Geometry: see drawing. Coordinates: mm, zero at the bounding-box minimum. A direction names the side the tool comes from. Coordinates: 2 decimals unless noted, no trailing zeros. Order: outer loops, then holes, each group sorted by start corner. A loop starts at its lowest first (then second) coordinate and runs counter-clockwise, first axis right, second up. Notation, with made-up numbers: (-31.75, 85.25) - (-13.75, 85.25) arc R13 ccw to (-13.75, 90.25) - close; hole circle Ø11 at (-4, 79). An arc over 180 degrees is marked (long way). Use a Markdown table: item, result. Add a question column.
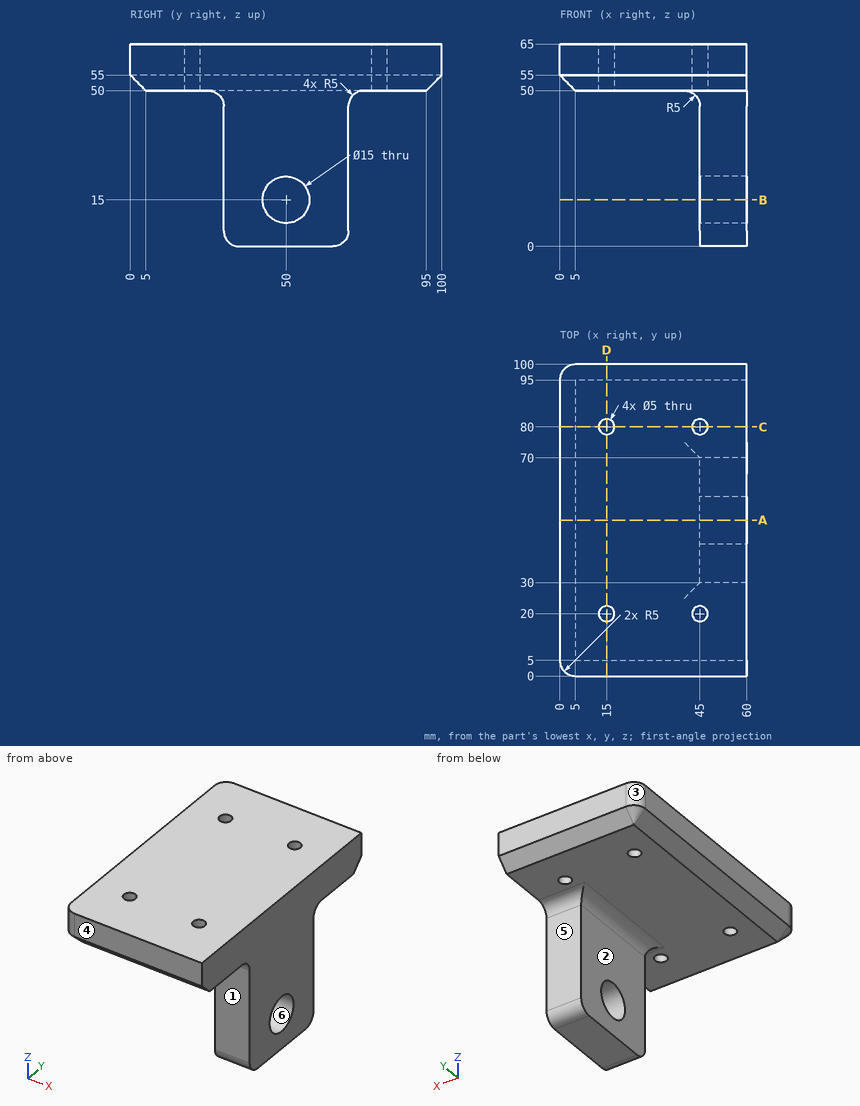
1) Cut plane D-D (x = 15). Return the cut outline in (y, z).
2) Cut plane C-C (y = 80). Return the cut outline in (x, z).
3) Cut plane B-B (z = 15). Return the cut outline in (x, y), and give its area (3 significant figures).
4) Material intervals for L1, parallel to Y at x = 15, z = 56.75; L2, parallel to Z at x = 56, y = 14.5; L3, parallel to Y at x = 49, z = 33.5, sorted ascending.
5) Reachability of the marked faces 1, 2 and 3 from +Z, -Z, +X, -X, +Y, -Y: full face, straight path, thin tool, end or side. Return the list, or none.
6) Contact query for flat-ended pins moving along their axis: P1, Ø2, axis at x = 46.5, y = 66.5, coming from the -Z side; P2, Ø4.5, axis at x = 49.5, z = 21.5, coming from the +Y side; P3, Ø1, axis at y = 58.5, z = 24, coming from the -X side; P4, Ø17, axis at y = 50, z = 15, coming from the +X side. Output: stop coordinate, or through.
7) Cut plane A-A (y = 50). Return the cut outline in (x, z), and give its area (3 significant figures).
8) Pull-direction query (Y, two-part tool) for the marked faces 4, 5 and 6; classes: pulls with the +Y half, pulls with the -Y half, needs draft (parallel to the pull), parting line crosses it, or undercut.
Computed:
| question | item | result |
|---|---|---|
| 1 | outline | (0, 55) - (5, 50) - (17.5, 50) - (17.5, 65) - (0, 65) - close; (22.5, 50) - (77.5, 50) - (77.5, 65) - (22.5, 65) - close; (82.5, 50) - (95, 50) - (100, 55) - (100, 65) - (82.5, 65) - close |
| 2 | outline | (0, 55) - (5, 50) - (12.5, 50) - (12.5, 65) - (0, 65) - close; (17.5, 50) - (42.5, 50) - (42.5, 65) - (17.5, 65) - close; (47.5, 50) - (60, 50) - (60, 65) - (47.5, 65) - close |
| 3 | outline | (45, 30) - (60, 30) - (60, 42.5) - (45, 42.5) - close; (45, 57.5) - (60, 57.5) - (60, 70) - (45, 70) - close |
| 3 | area | 375 mm2 |
| 4 | L1 | y = 0 to 17.5, 22.5 to 77.5, 82.5 to 100 |
| 4 | L2 | z = 50 to 65 |
| 4 | L3 | y = 30 to 70 |
| 5 | face 1 | -Z, +X, -X, -Y |
| 5 | face 2 | -Z, -X, +Y, -Y |
| 5 | face 3 | +Z, -Z, -X, +Y |
| 6 | P1 | stops at z = 0.03 |
| 6 | P2 | stops at y = 70 |
| 6 | P3 | stops at x = 45 |
| 6 | P4 | stops at x = 60 |
| 7 | outline | (0, 55) - (5, 50) - (40, 50) arc R5 cw to (45, 45) - (45, 22.5) - (60, 22.5) - (60, 65) - (0, 65) - close; (45, 0) - (60, 0) - (60, 7.5) - (45, 7.5) - close |
| 7 | area | 1,420 mm2 |
| 8 | face 4 | pulls with the -Y half |
| 8 | face 5 | pulls with the +Y half |
| 8 | face 6 | undercut |
